Read the model definition and answer for the solid it produces. Units are mm, in the model's axes. Give positions to 0.01 mm unless a question says otherwise; leave off trailing zeros.
```python
from build123d import *

# Parameters (mm, degrees)
SKETCH_2_R      = 2.5
EXTRUDE_1_DEPTH = 1800


with BuildPart() as part:
    # 草图2 → 凸台-拉伸1 (new body)
    with BuildSketch(Plane.XY):
        Polygon((-18.1, 37), (-18.1, 40), (-33, 40), (-33, 2.049564589), (-30, 2.049564589), (-30, 6.348214799), (-27.5, 6.348214799), (-27.5, 3.593219783), (-24, 3.593219783), (-24, 1.376590931), (-22.4, 1.376590931), (-22.4, -1.376590931), (-24, -1.376590931), (-24, -3.593219783), (-27.5, -3.593219783), (-27.5, -6.348214799), (-30, -6.348214799), (-30, -2.049564589), (-33, -2.049564589), (-33, -9.06837916), (-30.729793093, -9.06837916), (-30.729793093, -7.473013176), (-29.144133649, -7.473013176), (-29.144133649, -9.06837916), (-27.8, -9.06837916), (-27.8, -10.56837916), (-27.8, -12.06837916), (-29.144133649, -12.06837916), (-29.144133649, -13.663745144), (-30.729793093, -13.663745144), (-30.729793093, -12.06837916), (-33, -12.06837916), (-33, -40), (-12.5, -40), (-12.5, -17), (12.5, -17), (12.5, -40), (33, -40), (33, -12.06837916), (30.729793093, -12.06837916), (30.729793093, -13.663745144), (29.144133649, -13.663745144), (29.144133649, -12.06837916), (27.8, -12.06837916), (27.8, -10.56837916), (27.8, -9.06837916), (29.144133649, -9.06837916), (29.144133649, -7.473013176), (30.729793093, -7.473013176), (30.729793093, -9.06837916), (33, -9.06837916), (33, -2.049564589), (30, -2.049564589), (30, -6.348214799), (27.5, -6.348214799), (27.5, -3.593219783), (24, -3.593219783), (24, -1.376590931), (22.4, -1.376590931), (22.4, 1.376590931), (24, 1.376590931), (24, 3.593219783), (27.5, 3.593219783), (27.5, 6.348214799), (30, 6.348214799), (30, 2.049564589), (33, 2.049564589), (33, 40), (18.1, 40), (18.1, 37), (22.1, 37), (22.1, 34.5), (20.1, 34.5), (20.1, 31), (17.5, 31), (17.5, 29.4), (12.5, 29.4), (12.5, 31), (9.9, 31), (9.9, 34.5), (7.9, 34.5), (7.9, 37), (11.9, 37), (11.9, 40), (-11.9, 40), (-11.9, 37), (-7.9, 37), (-7.9, 34.5), (-9.9, 34.5), (-9.9, 31), (-12.5, 31), (-12.5, 29.4), (-17.5, 29.4), (-17.5, 31), (-20.1, 31), (-20.1, 34.5), (-22.1, 34.5), (-22.1, 37), align=None)
        with Locations((-27.8, -33.5)):
            Circle(SKETCH_2_R, mode=Mode.SUBTRACT)
        Polygon((-20.943121928, -13.45406673), (-20.943121928, -8.11004262), (-15.8, -15.86033199), (-15.8, -31.360910729), (-24, -31.360910729), (-24, -25.86703472), (-26.644243735, -25.86703472), (-26.644243735, -13.45406673), align=None, mode=Mode.SUBTRACT)
        with Locations((27.8, -33.5)):
            Circle(SKETCH_2_R, mode=Mode.SUBTRACT)
        Polygon((24, -25.86703472), (24, -31.360910729), (15.8, -31.360910729), (15.8, -15.86033199), (20.943121928, -8.11004262), (20.943121928, -13.45406673), (26.644243735, -13.45406673), (26.644243735, -25.86703472), align=None, mode=Mode.SUBTRACT)
        with Locations((-27.8, 33.5)):
            Circle(SKETCH_2_R, mode=Mode.SUBTRACT)
        Polygon((-24.000227571, 17.552802839), (-24.000227571, 21.788095294), (-17.932238887, 21.788095294), (-17.932238887, 24.712463894), (-10.638888278, 24.712463894), (-10.638888278, 28.169211595), (-4.9, 28.169211595), (-4.9, 37), (4.9, 37), (4.9, 28.169211595), (10.638888278, 28.169211595), (10.638888278, 24.712463894), (17.932238887, 24.712463894), (17.932238887, 21.788095294), (24.000227571, 21.788095294), (24.000227571, 17.552802839), (20.143121928, 17.552802839), (20.143121928, 14.174652905), (17.932238887, 14.174652905), (17.932238887, -5.752091446), (12.045824189, -14), (0, -14), (-12.045824189, -14), (-17.932238887, -5.752091446), (-17.932238887, 14.174652905), (-20.143121928, 14.174652905), (-20.143121928, 17.552802839), align=None, mode=Mode.SUBTRACT)
        with Locations((27.8, 33.5)):
            Circle(SKETCH_2_R, mode=Mode.SUBTRACT)
    extrude(amount=EXTRUDE_1_DEPTH)


solid = part.part
```
Item 1: Each of these flat-tipped pins is pushed along its axis until it touches: pin 1 Ø8 at (y, z) = (0, 1244) entering from +X; pin 2 Ø1.2 at (x, z) = (9, 900) entering from -Y; pin 3 Ø1 at (y, z) = (-1.5, 1083) entering from -X. Where does it stop, or does it pass through?
Result set:
pin 1: stops at x = 33
pin 2: stops at y = -17
pin 3: stops at x = -24
Item 2: Section A-A (z = 656) is taken. Give the number of separate pieces and of enclosed holes in the cut face, and give its area (3 significant figures).
Result set:
separate pieces: 1
enclosed holes: 7
area: 2,300 mm2
Item 3: Find the intervals of material crossed by line 1 along X through (y, z) = (-34, 357); line 2 along Y through (x, z) = (-28, 107.5); line 3 along Y through (x, z) = (-27, 462), in increasing order.
Result set:
line 1: x = -33 to -30.25, -25.35 to -12.5, 12.5 to 25.35, 30.25 to 33
line 2: y = -40 to -35.99, -31.01 to -12.07, -9.07 to -6.35, 6.35 to 31.01, 35.99 to 40
line 3: y = -40 to -35.87, -31.13 to -3.59, 3.59 to 31.13, 35.87 to 40
